Geometry: final body of the model. Coordinates: model frame, mm. Give positions to 0.01 mm unless a question says otherwise; leave off trailing zeros. Loops run counter-clockwise (first coordinate to the right, second up) from the corner with the lowest first, then second, coordinate; pieces in that order, holes last.
from build123d import *

# Parameters (mm, degrees)
SKETCH_1_R          = 11.1
SKETCH_1_R_2        = 10.5
EXTRUDE_1_DEPTH     = 10
SKETCH_3_W          = 6
SKETCH_3_H          = 3.4
CUT_EXTRUDE_1_DEPTH = 1.5


with BuildPart() as part:
    # 草图1 → 凸台-拉伸1 (new body)
    with BuildSketch(Plane.XY):
        Circle(SKETCH_1_R)
        Circle(SKETCH_1_R_2, mode=Mode.SUBTRACT)
    extrude(amount=EXTRUDE_1_DEPTH)

    # 草图3 → 切除-拉伸1 (cut)
    with BuildSketch(Plane.ZY.offset(11.1)):
        with Locations((5, 0.014841624)):
            Rectangle(SKETCH_3_W, SKETCH_3_H)
    extrude(amount=-CUT_EXTRUDE_1_DEPTH, mode=Mode.SUBTRACT)


solid = part.part
Item 1: Ray query, probe 1 along Y at (x, z) = (0, 6.75); probe 2 along X at (y, z) = (6.75, 8); probe 3 along X at (y, z) = (0, 7.5). Return the intervals inside material, ascending.
Values follow:
probe 1: y = -11.1 to -10.5, 10.5 to 11.1
probe 2: x = -8.81 to -8.04, 8.04 to 8.81
probe 3: x = 10.5 to 11.1
Item 2: Draft query along X for faces 1 (the face through (10.6, 3.3, 4.9)), 2 (the face through (10, 3.2, 4.9)), 3 (the face through (10, -4, 0)). Return one class per face: +X half, -X half, draft (parallel to the pull), parting line (faces both ways), or undercut.
Values follow:
face 1: parting line
face 2: undercut
face 3: draft
Item 3: Section query C-C on y = -8.25. Return loops of the section in (x, z), plus the area to 3 significant figures.
Values follow:
outline: (-7.43, 0) - (-6.5, 0) - (-6.5, 10) - (-7.43, 10) - close; (6.5, 0) - (7.43, 0) - (7.43, 10) - (6.5, 10) - close
area: 18.6 mm2
Item 4: Section query A-A on y = 0. Return loops of the section in (x, z).
Values follow:
outline: (-11.1, 0) - (-10.5, 0) - (-10.5, 2) - (-11.1, 2) - close; (-11.1, 8) - (-10.5, 8) - (-10.5, 10) - (-11.1, 10) - close; (10.5, 0) - (11.1, 0) - (11.1, 10) - (10.5, 10) - close
Item 5: Section query D-D on z = 6.5. Return loops of the section in (x, y).
Values follow:
outline: (-10.97, -1.69) arc R11.1 ccw (long way) to (-10.97, 1.71) - (-10.36, 1.71) arc R10.5 cw (long way) to (-10.36, -1.69) - close
Item 6: Pin query (flat end, axial travel): pin 1 (0.5 mm diameter, centred on x = -10.5, z = 4.5, fed in from -Y); pin 2 (1 mm diameter, centred on y = 1, z = 7, fed in from +X); pin 3 (12 mm diameter, centred on x = -8.5, y = -8, fed in from -Z); pin 4 (1.5 mm diameter, centred on y = 2.5, z = 6.5, fed in from +X). Return the tip coordinate at first contact, or that it passes through.
Values follow:
pin 1: stops at y = -4.26
pin 2: stops at x = 11.09
pin 3: stops at z = 0
pin 4: stops at x = 10.96
Item 7: Section query B-B on x = 0. Return loops of the section in (y, z), plus the area to 3 significant figures.
Values follow:
outline: (-11.1, 0) - (-10.5, 0) - (-10.5, 10) - (-11.1, 10) - close; (10.5, 0) - (11.1, 0) - (11.1, 10) - (10.5, 10) - close
area: 12.0 mm2
